Study the drawing (mm; zero at the part's minimum x, y, z) and answer. A direction names the side the tool comes from. Coordinates: 2 decimals unless noted, no trailing zeros. Loops run counter-clockwise (first coordinate to the right, second up) from the corner with the lowest first, then second, coordinate; pieces in that order, holes last. Notation, with made-up numbers: (-15.5, 35.25) - (-11.5, 35.25) arc R24 ccw to (-11.5, 65.25) - close; hole circle Ø4 at (-28, 30.25). An arc over 180 degrees is marked (long way). Use one line per item in the form item = value.
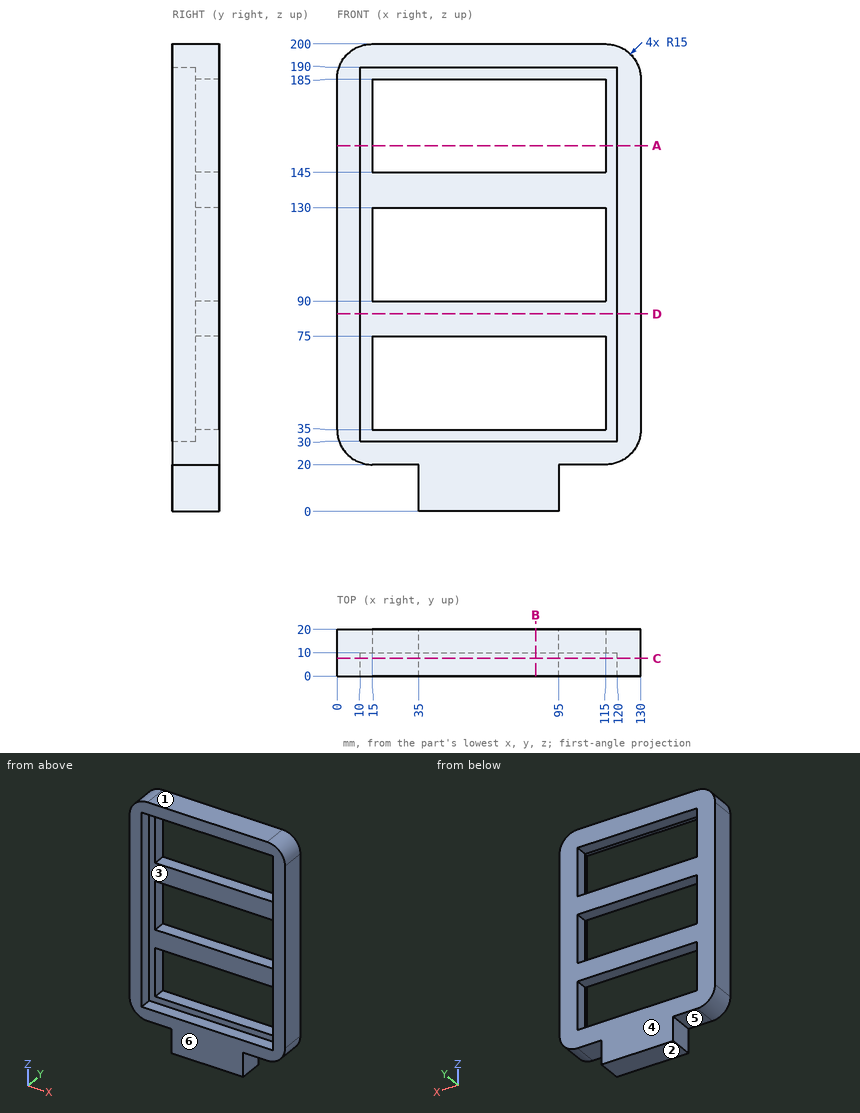
Item 1: Find the intervals of material crossed by L1, parallel to Z at x = 96, y = 13.75; L2, parallel to Z at x = 40, y = 16.75; L3, parallel to Z at x = 88, y = 9, in increasing order.
Results below:
L1 = 20 to 35, 75 to 90, 130 to 145, 185 to 200
L2 = 0 to 35, 75 to 90, 130 to 145, 185 to 200
L3 = 0 to 30, 190 to 200
Item 2: Each of these flat-tipped pins is pushed along its axis until it touches: P1, Ø6, axis at y = 10, z = 9.5, coming from the +X side; P2, Ø6, axis at y = 6, z = 15, coming from the -X side. Where does it stop, or does it pass through?
Results below:
P1 = 95
P2 = 35
Item 3: The part is cut by section D-D on z = 84.5. Give the vertices of the cut face in (x, y), plus the area to 3 significant figures.
Results below:
outline = (0, 0) - (10, 0) - (10, 10) - (120, 10) - (120, 0) - (130, 0) - (130, 20) - (0, 20) - close
area = 1,500 mm²
Item 4: The part is cut by section C-C on y = 7.5. Give the vertices of the cut face in (x, z).
Results below:
outline = (0, 35) arc R15 ccw to (15, 20) - (35, 20) - (35, 0) - (95, 0) - (95, 20) - (115, 20) arc R15 ccw to (130, 35) - (130, 185) arc R15 ccw to (115, 200) - (15, 200) arc R15 ccw to (0, 185) - close; hole (10, 30) - (120, 30) - (120, 190) - (10, 190) - close
Item 5: The part is cut by section A-A on z = 156.5. Give the vertices of the cut face in (x, y), plus the area to 3 significant figures.
Results below:
outline = (0, 0) - (10, 0) - (10, 10) - (15, 10) - (15, 20) - (0, 20) - close; (115, 10) - (120, 10) - (120, 0) - (130, 0) - (130, 20) - (115, 20) - close
area = 500 mm²
Item 6: Which of the six approach directions +Z, -Z, +X, -X, +Y, -Y give full straight-line access (tool end or side, diameter ignored) to the marked faces 5 and 6?
Results below:
face_5 = -Z, -X, +Y, -Y
face_6 = +Z, -Z, +X, -X, -Y
Item 7: For a pull along Z with two mould halves and no side action, classify the marked faces 1, 2, 3 and 4 as +Z half, -Z half, draft (parallel to the pull), parting line (faces both ways), or undercut.
Results below:
face_1 = +Z half
face_2 = -Z half
face_3 = undercut
face_4 = draft
Item 8: The part is cut by section B-B on x = 85. Give the vertices of the cut face in (y, z).
Results below:
outline = (0, 0) - (20, 0) - (20, 35) - (10, 35) - (10, 30) - (0, 30) - close; (0, 190) - (10, 190) - (10, 185) - (20, 185) - (20, 200) - (0, 200) - close; (10, 75) - (20, 75) - (20, 90) - (10, 90) - close; (10, 130) - (20, 130) - (20, 145) - (10, 145) - close
